Geometry check sheet. Reference: drawing and pictorial views, mm from the part's lowest x, y, z. A direction names the side the tool comes from. Give positions to 0.01 mm unless a question says otherwise; leave off trailing zeros. Order: outer loops, then holes, each group sorted by start corner. A loop starts at its lowest first (then second) coordinate and runs counter-clockwise, first axis right, second up.
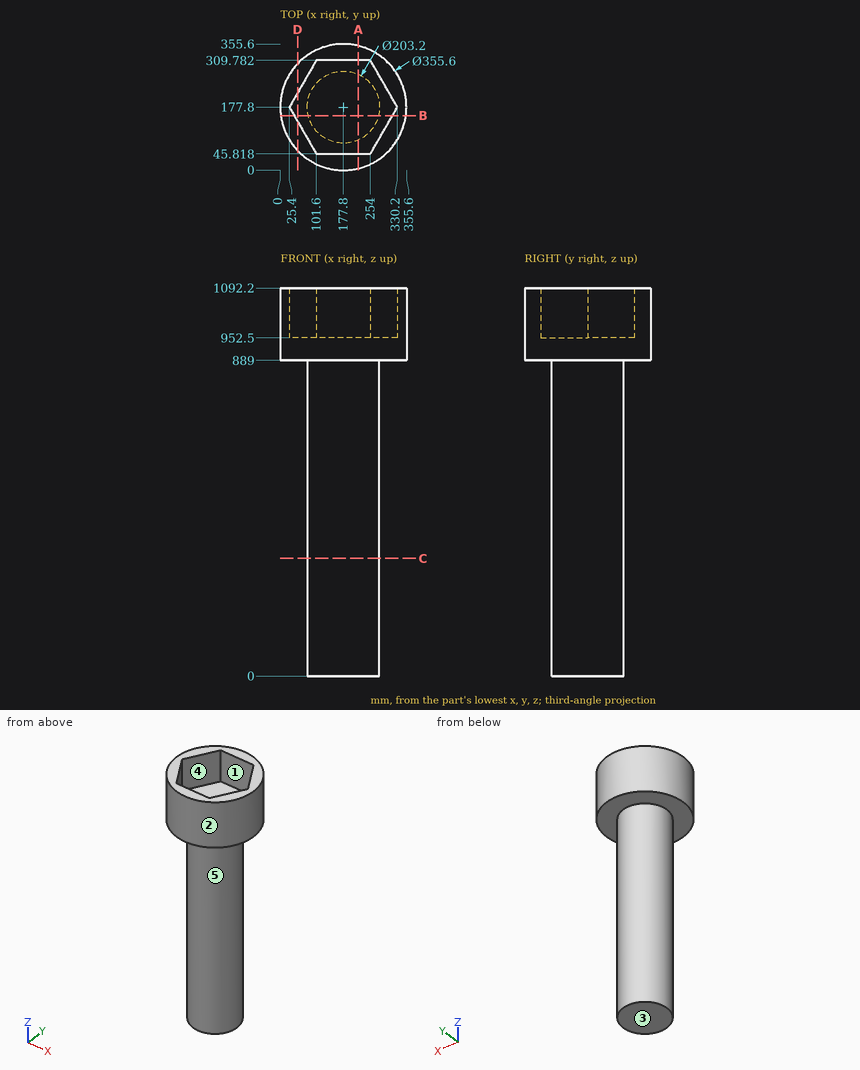
1) Section check B-B, the plane y = 154. Record the cut outline in (x, z), then the cut area to 3 significant figures.
Recorded:
outline: (1.6, 889) - (79.03, 889) - (79.03, 0) - (276.57, 0) - (276.57, 889) - (354, 889) - (354, 1092.2) - (316.46, 1092.2) - (316.46, 952.5) - (39.14, 952.5) - (39.14, 1092.2) - (1.6, 1092.2) - close
area: 208,000 mm2
2) Depth check by flat-ended pin: pin 1 Ø1 at (x, y) = (228.5, 83.5) entering from +Z; pin 2 Ø6 at (y, z) = (105.5, 328) entering from +X; pin 3 Ø4 at (x, y) = (54.5, 304.5) entering from -Z. Enter the tip coordinate at first touch or a pass-through.
Recorded:
pin 1: stops at z = 952.5
pin 2: stops at x = 252.1
pin 3: stops at z = 889
3) Material ranges on L1, parallel to Z at x = 79.5, y = 40; L2, parallel to Y at x = 311.5, z = 1038.5 (1 decimal); L3, parallel to X at y = 187.5, z = 1017 (1 decimal), recorded low to high.
Recorded:
L1: z = 889 to 1092.2
L2: y = 60.6 to 145.4, 210.2 to 295
L3: x = 0.3 to 31, 324.6 to 355.3
4) Set-up check for the marked faces 4 and 5: record each of +Z, -Z, +X, -X, +Y, -Y from which the full face is reachable in a straight line by a thin tool's end or side.
Recorded:
face 4: +Z
face 5: -Z
5) Section check A-A, the plane x = 220. Record the cut outline in (y, z), then the cut area to 3 significant figures.
Recorded:
outline: (5.08, 889) - (85.38, 889) - (85.38, 0) - (270.22, 0) - (270.22, 889) - (350.52, 889) - (350.52, 1092.2) - (309.78, 1092.2) - (309.78, 952.5) - (45.82, 952.5) - (45.82, 1092.2) - (5.08, 1092.2) - close
area: 198,000 mm2
6) Draft check along X on the marked faces 1, 2 and 3. Enter one of: +X half, -X half, draft (parallel to the pull), parting line (faces both ways), or undercut.
Recorded:
face 1: undercut
face 2: parting line
face 3: draft
7) Section check C-C, the plane z = 331. Record the cut outline in (x, y), then the cut area to 3 significant figures.
Recorded:
outline: circle Ø203.2 at (177.8, 177.8)
area: 32,400 mm2
8) Section check D-D, the plane x = 49. Record the cut outline in (y, z).
Recorded:
outline: (55.23, 889) - (300.37, 889) - (300.37, 1092.2) - (218.68, 1092.2) - (218.68, 952.5) - (136.92, 952.5) - (136.92, 1092.2) - (55.23, 1092.2) - close
